Source: CAD feature listing. Evaluate the final solid. Frame: model axes, mm. A direction names the side the tool comes from. Give positions to 0.01 mm unless a question says otherwise; leave off trailing zeros. Order: outer loops, then holes, each group sorted by start corner. A loop starts at its lowest first (then second) coordinate and runs counter-clockwise, first axis right, second up. Notation, with made-up numbers: (18, 32) -> (39, 32) arc R19 cw to (39, 63) -> close; hole circle Ø6 at (13.5, 56.5). An arc over 180 degrees is marked (long way). Use CSV: the item, a comma, the result in double quotes.
Solid Edge part; units mm, degrees
sketch "Sketch1" plane through (0, 0, 0) normal (0, -1, 0) x (1, 0, 0)
  circle A0 centre (0, 0) radius 30
  circle A1 centre (0, 0) radius 15
extrude "Protrusion1" add sketch "Sketch1" along normal mid plane 80
sketch "Sketch2" plane through (0, 0, 0) normal (0, 1, 0) x (-1, 0, 0)
  line L0 (-66, 0) -> (-13.6364, 26.7217)
  line L1 (-13.6364, 26.7217) -> (-30, 0)
  line L2 (-30, 0) -> (-66, 0)
extrude "ExtrudedProtrusion_2" add sketch "Sketch2" along normal mid plane 12
sketch "Sketch3" plane through (48, 0, 0) normal (0, 0, -1) x (0, 1, 0)
  line L0 (-30, -28.3201) -> (-30, 18)
  line L1 (-30, 18) -> (0, 18)
  line L2 (0, 18) -> (30, 18)
  line L3 (30, 18) -> (30, -28.3201)
  line L4 (30, -28.3201) -> (-30, -28.3201)
extrude "ExtrudedProtrusion_3" add sketch "Sketch3" along normal blind 20
sketch "Sketch4" plane through (66, 0, -10) normal (1, 0, 0) x (0, 0, -1)
  line L0 (-10, -30) -> (30, -30)
  line L1 (-10, 30) -> (-10, -30)
  line L2 (30, 30) -> (-10, 30)
  arc A0 (30, 30) -> (30, -30) centre (30, 0) cw
extrude "ExtrudedProtrusion_4" add sketch "Sketch4" against normal blind 20
sketch "Sketch5" plane through (48, -18, -40) normal (0, 0, 1) x (0, -1, 0)
  line L0 (2, 58) -> (12, 18)
  line L1 (12, 18) -> (-8, 18)
  line L2 (-8, 18) -> (-8, 58)
  line L3 (-8, 58) -> (2, 58)
revolve "RevolvedProtrusion1" add sketch "Sketch5" angle 360 about axis through (66, 0, -40) along (1, 0, 0)
sketch "Sketch6" plane through (46, 0, -45) normal (-1, 0, 0) x (0, -1, 0)
  circle A0 centre (0, 5) radius 10
extrude "Cutout1" cut sketch "Sketch6" against normal up to vertex (60 mm away)
1. Mould query, pull axis Y, two halves, no side actions, for faces 1 (the flat face through (49, -30, -15)), 2 (the cylindrical face through (76.42, 2.17, -30.24)), 3 (the flat face through (66, 0, -6)). Classes: released by +Y, released by -Y, zero draft, split by the parting line, or undercut.
Answer below:
face 1,"released by -Y"
face 2,"undercut"
face 3,"zero draft"
2. Section query C-C on x = 61. Return loops of the section in (y, z), plus the area to 3 significant figures.
Answer below:
outline,"(-30, -40) arc R30 ccw to (30, -40) -> (30, 0) -> (6, 0) -> (6, 2.55) -> (-6, 2.55) -> (-6, 0) -> (-30, 0) -> close; hole circle Ø20 at (0, -40)"
area,"3,530 mm²"
3. Section query B-B on x = 0. Return loops of the section in (y, z), plus the area to 3 significant figures.
Answer below:
outline,"(-40, -30) -> (40, -30) -> (40, -15) -> (-40, -15) -> close; (-40, 15) -> (40, 15) -> (40, 30) -> (-40, 30) -> close"
area,"2,400 mm²"
4. Section query D-D on x = -21. Return loops of the section in (y, z).
Answer below:
outline,"(-40, -21.42) -> (40, -21.42) -> (40, 21.42) -> (-40, 21.42) -> close"
5. Section query A-A on y = 0. Count the separate pieces of the cut face and the enclosed holes in it, plus the area to 3 significant figures.
Answer below:
separate pieces,"2"
enclosed holes,"1"
area,"5,080 mm²"
6. Pin query (flat end, axial travel): P1, Ø3, axis at x = 38, y = 30, coming from the +Z side; P2, Ø12, axis at x = 37.5, z = -15.5, coming from the -Y side; P3, Ø4, axis at x = 89, y = 2.5, coming from the +Z side. Return the tip coordinate at first contact, or that it passes through.
Answer below:
P1,"stops at z = 0"
P2,"stops at y = -30"
P3,"stops at z = -15.35"
7. Ray query, line 1 along Z through (x, y) = (0, 15); line 2 along Z through (x, y) = (60, 0); line 3 along Y through (x, z) = (36.5, 10). Return the intervals inside material, ascending.
Answer below:
line 1,"z = -30 to -15, 15 to 30"
line 2,"z = -70 to -50, -30 to 3.06"
line 3,"y = -6 to 6"
8. Access query for faces 4 (the flat face through (34, 0, -20)), 5 (the flat face through (40, 6, 7)), 6 (the cylindrical face through (-29.97, -0.56, 1.32)), 7 (the flat face through (48, -18, 0)). Directions: +Z, -Z, +X, -X, +Y, -Y. A direction counts if a zero-diameter tool reaches every point of the face in a straight line with its end or side. Return the directions, or none.
Answer below:
face 4,"-Z, +Y, -Y"
face 5,"+Z, +X, +Y"
face 6,"none"
face 7,"+Z, +X, -Y"
